```python
from build123d import *

# Parameters (mm, degrees)
BOSS_EXTRUDE1_DEPTH             = 10.16
SKETCH6_W                       = 10.16
SKETCH6_H                       = 1.27
BOSS_EXTRUDE3_DEPTH             = 3.81
SKETCH8_W                       = 4.826
SKETCH8_H                       = 0.762
CUT_EXTRUDE1_DEPTH              = 2.2352
SKETCH5_W                       = 4.826
SKETCH5_H                       = 0.762
CUT_EXTRUDE2_DEPTH              = 2.2352
SKETCH17_R                      = 1.27
CUT_EXTRUDE3_DEPTH              = 2.54
F_6_32_TAPPED_HOLE1_D           = 2.7051
F_6_32_TAPPED_HOLE1_DEPTH       = 9.398
F_6_32_TAPPED_HOLE1_CSINK_D     = 4.7752
F_6_32_TAPPED_HOLE1_CSINK_ANGLE = 100
F_6_32_TAPPED_HOLE1_TIP         = 0.81269403


with BuildPart() as part:
    # Sketch1 → Boss-Extrude1 (new body)
    with BuildSketch(Plane.XY):
        Polygon((-22.483233333, 11.63955), (-22.483233333, -18.84045), (-18.673233333, -18.84045), (-18.673233333, -20.11045), (-23.753233333, -20.11045), (-23.753233333, 11.63955), align=None)
    extrude(amount=BOSS_EXTRUDE1_DEPTH)

    # Sketch6 → Boss-Extrude3 (add)
    with BuildSketch(Plane(origin=(-22.483233333, 0, 0), x_dir=(0, 0, -1), z_dir=(1, 0, 0))):
        with Locations((-5.08, 2.87655)):
            Rectangle(SKETCH6_W, SKETCH6_H)
    extrude(amount=BOSS_EXTRUDE3_DEPTH)

    # Sketch8 → Cut-Extrude1 (cut)
    with BuildSketch(Plane(origin=(-18.673233333, 0, 0), x_dir=(0, 0, -1), z_dir=(1, 0, 0))):
        with Locations((-5.08, 2.87655)):
            Rectangle(SKETCH8_W, SKETCH8_H)
    extrude(amount=-CUT_EXTRUDE1_DEPTH, mode=Mode.SUBTRACT)

    # Sketch5 → Cut-Extrude2 (cut)
    with BuildSketch(Plane(origin=(-18.673233333, 0, 0), x_dir=(0, 0, -1), z_dir=(1, 0, 0))):
        with Locations((-5.08, -19.47545)):
            Rectangle(SKETCH5_W, SKETCH5_H)
    extrude(amount=-CUT_EXTRUDE2_DEPTH, mode=Mode.SUBTRACT)

    # Sketch17 → Cut-Extrude3 (cut)
    with BuildSketch(Plane(origin=(-22.483233333, 0, 0), x_dir=(0, 0, -1), z_dir=(1, 0, 0))):
        with Locations((-5.08, -7.084396388)):
            Circle(SKETCH17_R)
    extrude(amount=-CUT_EXTRUDE3_DEPTH, mode=Mode.SUBTRACT)

    # #6-32 Tapped Hole1
    with Locations(Plane.ZY.offset(23.753233333)):
        with Locations((5.111682079, 8.84555)):
            CounterSinkHole(F_6_32_TAPPED_HOLE1_D / 2, F_6_32_TAPPED_HOLE1_CSINK_D / 2, depth=F_6_32_TAPPED_HOLE1_DEPTH, counter_sink_angle=F_6_32_TAPPED_HOLE1_CSINK_ANGLE)
            with Locations((0, 0, -(F_6_32_TAPPED_HOLE1_DEPTH + F_6_32_TAPPED_HOLE1_TIP / 2))):  # 118° drill point
                Cone(0, F_6_32_TAPPED_HOLE1_D / 2, F_6_32_TAPPED_HOLE1_TIP, mode=Mode.SUBTRACT)


solid = part.part
```
Geometry check sheet. Reference: the model listing, model coordinates, mm. A direction names the side the tool comes from. Give positions to 0.01 mm unless a question says otherwise; leave off trailing zeros. Order: outer loops, then holes, each group sorted by start corner. A loop starts at its lowest first (then second) coordinate and runs counter-clockwise, first axis right, second up.
1. Section check B-B, the plane x = -21.45. Enter the section's corners in (y, z), and give its area (3 significant figures).
2. Section check D-D, the plane x = -23.4. Enter the section's corners in (y, z), and give its area (3 significant figures).
3. Thickness scan on L1, parallel to Y at x = -21.55, z = 5.5; L2, parallel to Y at x = -22.9, z = 4.5; L3, parallel to Y at x = -23.3, z = 5.08. Record the ranges inside material, lowest first.
4. Access from +Z, -Z, +X, -X, +Y, -Y to the whole of each face (thin tool, end or side, straight path). Record for faces 1 (the face through (-22.483, 7, 5)), 2 (the face through (-21, 2.242, 5)), 3 (the face through (-20, 2.496, 5)).
5. Gauge pin test, flat ends, axial feed: pin 1 Ø1.5 at (y, z) = (-7.08, 5.08) entering from -X; pin 2 Ø1.8 at (x, z) = (-20, 5.5) entering from +Y; pin 3 Ø6 at (y, z) = (-7, 8) entering from +X; pin 4 Ø3 at (y, z) = (8.85, 5.11) entering from -X. Record the tip position at first contact, or that the pin passes through.
6. Section check C-C, the plane z = 9.25. Enter the section's corners in (x, y), and give its area (3 significant figures).
7. Section check A-A, the plane x = -20. Enter the section's corners in (y, z), and give its area (3 significant figures).
8. Release check for a two-part mould opening along Z. For faces 4 (the face through (-23, -5, 10.16)), 5 (the face through (-20, 3.258, 5)), 6 (the face through (-22.681, 7.525, 5.405)), 7 (the face through (-22.483, -8.2, 3.9)) record: pulls with the +Z half, pulls with the -Z half, needs draft (parallel to the pull), parting line crosses it, or undercut.
Values follow:
1. outline: (-20.11, 0) - (-18.84, 0) - (-18.84, 10.16) - (-20.11, 10.16) - close; (2.24, 0) - (3.51, 0) - (3.51, 10.16) - (2.24, 10.16) - close
1. area: 25.8 mm2
2. outline: (-20.11, 0) - (11.64, 0) - (11.64, 10.16) - (-20.11, 10.16) - close; hole circle Ø2.54 at (-7.08, 5.08); hole circle Ø3.93 at (8.85, 5.11)
2. area: 305 mm2
3. L1: y = -20.11 to -18.84, 2.24 to 3.51
3. L2: y = -20.11 to -8.21, -5.95 to 7.62, 10.07 to 11.64
3. L3: y = -20.11 to -8.35, -5.81 to 7, 10.69 to 11.64
4. face 1: +Z, -Z, +X, +Y
4. face 2: +Z, -Z, +X
4. face 3: +X
5. pin 1: passes through
5. pin 2: stops at y = 3.51
5. pin 3: stops at x = -22.48
5. pin 4: stops at x = -23.01
6. outline: (-23.75, -20.11) - (-18.67, -20.11) - (-18.67, -18.84) - (-22.48, -18.84) - (-22.48, 2.24) - (-18.67, 2.24) - (-18.67, 3.51) - (-22.48, 3.51) - (-22.48, 11.64) - (-23.75, 11.64) - close
6. area: 50.0 mm2
7. outline: (-20.11, 0) - (-18.84, 0) - (-18.84, 10.16) - (-20.11, 10.16) - close; (2.24, 0) - (3.51, 0) - (3.51, 10.16) - (2.24, 10.16) - close; hole (-19.86, 2.67) - (-19.09, 2.67) - (-19.09, 7.49) - (-19.86, 7.49) - close; hole (2.5, 2.67) - (3.26, 2.67) - (3.26, 7.49) - (2.5, 7.49) - close
7. area: 18.5 mm2
8. face 4: pulls with the +Z half
8. face 5: undercut
8. face 6: undercut
8. face 7: needs draft
